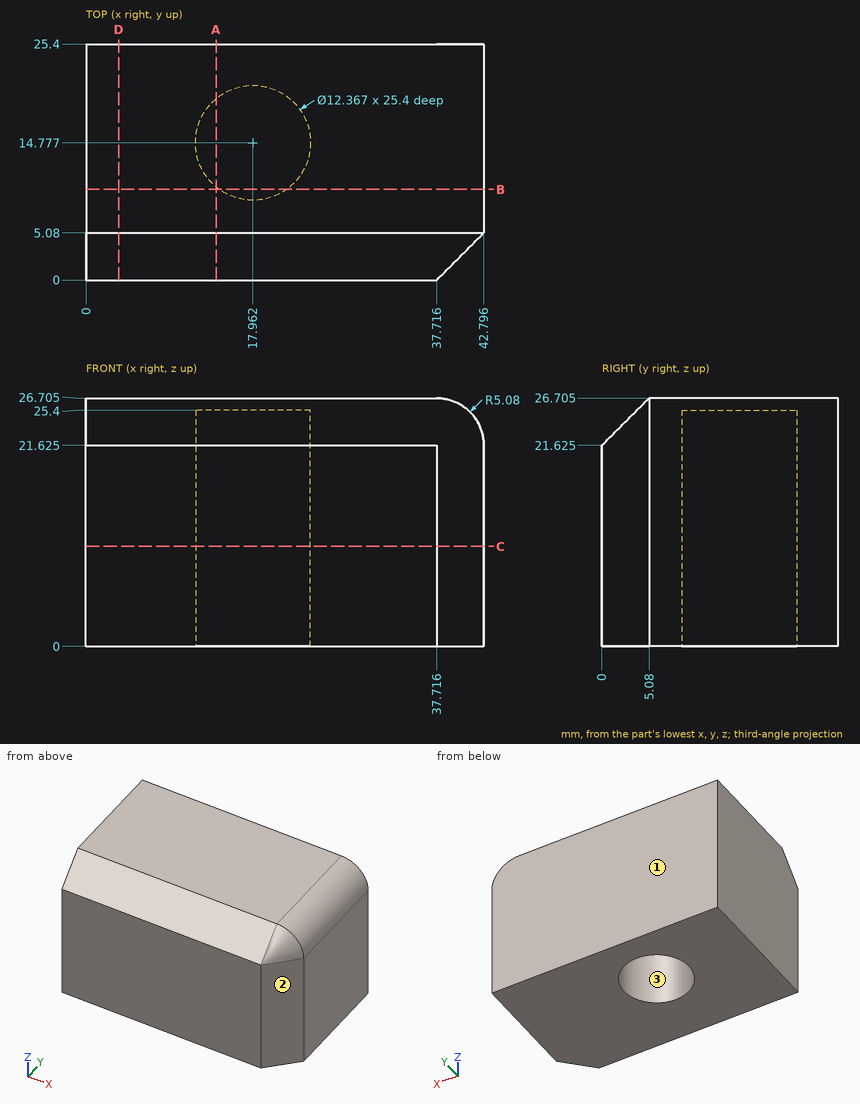
Design review of the part shown in the three views and the two pictorial views. Dimensions are in mm from the part's minimum x, y and z. Round coordinates to 2 decimals unless told otherwise and drop trailing zeros. Loops run counter-clockwise (first coordinate to the right, second up) from the corner with the lowest first, then second, coordinate; pieces in that order, holes last. Notation, with made-up numbers: (71, 52) - (90, 52) arc R13 cw to (90, 68) - close; hole circle Ø11 at (-19, -39). An arc over 180 degrees is marked (long way). Use one line per item in the form item = value.
1) We need section B-B on y = 9.75. Write out the cut boundary in (x, z) (1 decimal).
Solutions:
outline = (0, 0) - (14.4, 0) - (14.4, 25.4) - (21.6, 25.4) - (21.6, 0) - (42.8, 0) - (42.8, 21.6) arc R5.1 ccw to (37.7, 26.7) - (0, 26.7) - close
2) Mouldability with a two-part tool opening along X and no side actions: class the marked faces 1, 2 and 3 as pulls with the +X half, pulls with the -X half, needs draft (parallel to the pull), parting line crosses it, or undercut.
Solutions:
face_1 = needs draft
face_2 = pulls with the +X half
face_3 = undercut
3) Clearance check with flat-ended pins moving along their axes: P1, Ø10, axis at x = 15, y = 12.5, coming from the -Z side; P2, Ø2, axis at x = 14.5, y = 13.5, coming from the -Z side. State where each tip first meets the part, or that it passes through.
Solutions:
P1 = 0
P2 = 25.4
4) We need section D-D on x = 3.5. Write out the cut boundary in (y, z) (1 decimal), then the cut area to 3 significant figures.
Solutions:
outline = (0, 0) - (25.4, 0) - (25.4, 26.7) - (5.1, 26.7) - (0, 21.6) - close
area = 665 mm2
5) We need section A-A on x = 14. Write out the cut boundary in (y, z) (1 decimal), then the cut area to 3 significant figures.
Solutions:
outline = (0, 0) - (10, 0) - (10, 25.4) - (19.5, 25.4) - (19.5, 0) - (25.4, 0) - (25.4, 26.7) - (5.1, 26.7) - (0, 21.6) - close
area = 424 mm2
6) We need section C-C on z = 10.75. Write out the cut boundary in (x, y) (1 decimal).
Solutions:
outline = (0, 0) - (37.7, 0) - (42.8, 5.1) - (42.8, 25.4) - (0, 25.4) - close; hole circle Ø12.4 at (18, 14.8)
7) Wall thickness on probe 1 along Y at (x, z) = (19.5, 4.25) (1 decimal); probe 2 along Z at (x, y) = (12.5, 13.75) (1 decimal); probe 3 along X at (y, z) = (11.25, 4.25) (1 decimal): over which ranges is each line inside the solid? List them lowest first.
Solutions:
probe_1 = 0 to 8.8, 20.8 to 25.4
probe_2 = 25.4 to 26.7
probe_3 = 0 to 12.9, 23 to 42.8
